CAD build for the part. Positions are in the model's coordinates, mm. A direction names the side the tool comes from. Round coordinates to 2 decimals unless told otherwise and drop trailing zeros. Order: outer loops, then holes, each group sorted by start corner. A loop starts at its lowest first (then second) coordinate and runs counter-clockwise, first axis right, second up. Notation, with made-up numbers: (-24, 77) - (14, 77) arc R14 cw to (14, 82) - close; hole circle Ø10 at (80.25, 87). An arc over 180 degrees is marked (long way). Write item = value, one per line.
from build123d import *

# Parameters (mm, degrees)
BOSS_EXTRUDE1_DEPTH = 20
SKETCH2_W           = 40
SKETCH2_H           = 40
BOSS_EXTRUDE2_DEPTH = 80
SKETCH3_W           = 40
SKETCH3_H           = 60
SKETCH3_H_2         = 40
SKETCH3_W_2         = 60
BOSS_EXTRUDE3_DEPTH = 20
SKETCH5_R           = 2.75
CUT_EXTRUDE1_DEPTH  = 167
FILLET1_R           = 25
FILLET2_R           = 15
SKETCH6_W           = 5
SKETCH6_H           = 10
SKETCH6_W_2         = 10
SKETCH6_H_2         = 5
BOSS_EXTRUDE4_DEPTH = 10
CUT_EXTRUDE2_DEPTH  = 10
CUT_EXTRUDE3_DEPTH  = 10
SKETCH9_W           = 10
SKETCH9_H           = 5
SKETCH9_W_2         = 5
SKETCH9_H_2         = 10
BOSS_EXTRUDE5_DEPTH = 10
CUT_EXTRUDE4_DEPTH  = 10
CUT_EXTRUDE5_DEPTH  = 10
FILLET4_R           = 3


with BuildPart() as part:
    # Sketch1 → Boss-Extrude1 (new body)
    with BuildSketch(Plane.XY):
        Polygon((100, 380), (100, 340), (40, 340), (40, 280), (0, 280), (0, 380), align=None)
    extrude(amount=BOSS_EXTRUDE1_DEPTH)

    # Sketch2 → Boss-Extrude2 (add)
    with BuildSketch(Plane.XY.offset(20)):
        with Locations((20, 360)):
            Rectangle(SKETCH2_W, SKETCH2_H)
    extrude(amount=BOSS_EXTRUDE2_DEPTH)

    # Sketch3 → Boss-Extrude3 (add)
    with BuildSketch(Plane.XY.offset(100)):
        with Locations((20, 310)):
            Rectangle(SKETCH3_W, SKETCH3_H)
        with Locations((20, 360)):
            Rectangle(SKETCH3_W, SKETCH3_H_2)
        with Locations((70, 360)):
            Rectangle(SKETCH3_W_2, SKETCH3_H_2)
    extrude(amount=BOSS_EXTRUDE3_DEPTH)

    # Sketch5 → Cut-Extrude1 (cut)
    with BuildSketch(Plane.XY.offset(120)):
        with Locations((55, 360)):
            Circle(SKETCH5_R)
        with BuildLine():
            ThreePointArc((82.25, 360), (85, 357.25), (87.75, 360))
            Line((87.75, 360), (82.25, 360))
        make_face()
        with BuildLine():
            Line((82.25, 360), (87.75, 360))
            ThreePointArc((87.75, 360), (85, 362.75), (82.25, 360))
        make_face()
        with Locations((20, 325)):
            Circle(SKETCH5_R)
        with BuildLine():
            ThreePointArc((22.75, 295), (21.944543648, 296.944543648), (20, 297.75))
            Line((20, 297.75), (20, 292.25))
            ThreePointArc((20, 292.25), (21.944543648, 293.055456352), (22.75, 295))
        make_face()
        with BuildLine():
            Line((20, 292.25), (20, 297.75))
            ThreePointArc((20, 297.75), (17.25, 295), (20, 292.25))
        make_face()
    extrude(amount=-CUT_EXTRUDE1_DEPTH, mode=Mode.SUBTRACT)

    # Fillet1
    # the kernel refuses this fillet: 25 mm, written as the material it takes off along each edge
    with BuildSketch(Plane(origin=(40, 340, 20), x_dir=(0, 1, 0), z_dir=(0, 0, 1))) as fillet1_piece_1:
        with BuildLine():
            CenterArc((FILLET1_R, FILLET1_R), FILLET1_R, 180, 90)
            Line((0, FILLET1_R), (0, 0))
            Line((0, 0), (FILLET1_R, 0))
        make_face()
    extrude(amount=80, mode=Mode.SUBTRACT)

    # Fillet2
    fillet2_edges = [part.edges().sort_by_distance(p)[0] for p in [
        (100, 340, 10),
        (40, 340, 10),
        (40, 280, 10),
        (40, 280, 110),
        (40, 340, 110),
        (100, 340, 110),
    ]]
    fillet(fillet2_edges, radius=FILLET2_R)

    # Sketch6 → Boss-Extrude4 (add)
    with BuildSketch(Plane.XY.offset(20)):
        with Locations((2.5, 310)):
            Rectangle(SKETCH6_W, SKETCH6_H)
        with Locations((70, 377.5)):
            Rectangle(SKETCH6_W_2, SKETCH6_H_2)
    extrude(amount=BOSS_EXTRUDE4_DEPTH)

    # Sketch7 → Cut-Extrude2 (cut)
    with BuildSketch(Plane.XZ.offset(-375)):
        with BuildLine():
            ThreePointArc((71.75, 25), (71.237436867, 26.237436867), (70, 26.75))
            Line((70, 26.75), (70, 23.25))
            ThreePointArc((70, 23.25), (71.237436867, 23.762563133), (71.75, 25))
        make_face()
        with BuildLine():
            Line((70, 23.25), (70, 26.75))
            ThreePointArc((70, 26.75), (68.25, 25), (70, 23.25))
        make_face()
    extrude(amount=-CUT_EXTRUDE2_DEPTH, mode=Mode.SUBTRACT)

    # Sketch8 → Cut-Extrude3 (cut)
    with BuildSketch(Plane(origin=(5, 0, 0), x_dir=(0, 0, -1), z_dir=(1, 0, 0))):
        with BuildLine():
            ThreePointArc((-23.25, 310), (-25, 311.75), (-26.75, 310))
            Line((-26.75, 310), (-23.25, 310))
        make_face()
        with BuildLine():
            Line((-23.25, 310), (-26.75, 310))
            ThreePointArc((-26.75, 310), (-25, 308.25), (-23.25, 310))
        make_face()
    extrude(amount=-CUT_EXTRUDE3_DEPTH, mode=Mode.SUBTRACT)

    # Sketch9 → Boss-Extrude5 (add)
    with BuildSketch(Plane(origin=(0, 0, 100), x_dir=(-1, 0, 0), z_dir=(0, 0, -1))):
        with Locations((-70, 377.5)):
            Rectangle(SKETCH9_W, SKETCH9_H)
        with Locations((-2.5, 310)):
            Rectangle(SKETCH9_W_2, SKETCH9_H_2)
    extrude(amount=BOSS_EXTRUDE5_DEPTH)

    # Sketch10 → Cut-Extrude4 (cut)
    with BuildSketch(Plane(origin=(5, 0, 0), x_dir=(0, 0, -1), z_dir=(1, 0, 0))):
        with BuildLine():
            ThreePointArc((-96.75, 310), (-95, 308.25), (-93.25, 310))
            Line((-93.25, 310), (-96.75, 310))
        make_face()
        with BuildLine():
            Line((-96.75, 310), (-93.25, 310))
            ThreePointArc((-93.25, 310), (-95, 311.75), (-96.75, 310))
        make_face()
    extrude(amount=-CUT_EXTRUDE4_DEPTH, mode=Mode.SUBTRACT)

    # Sketch11 → Cut-Extrude5 (cut)
    with BuildSketch(Plane.XZ.offset(-375)):
        with BuildLine():
            ThreePointArc((71.75, 95), (71.237436867, 96.237436867), (70, 96.75))
            Line((70, 96.75), (70, 93.25))
            ThreePointArc((70, 93.25), (71.237436867, 93.762563133), (71.75, 95))
        make_face()
        with BuildLine():
            Line((70, 93.25), (70, 96.75))
            ThreePointArc((70, 96.75), (68.25, 95), (70, 93.25))
        make_face()
    extrude(amount=-CUT_EXTRUDE5_DEPTH, mode=Mode.SUBTRACT)

    # Fillet4
    fillet4_edges = [part.edges().sort_by_distance(p)[0] for p in [
        (2.5, 315, 30),
        (2.5, 305, 20),
        (2.5, 305, 30),
        (2.5, 315, 20),
        (75, 377.5, 30),
        (65, 377.5, 20),
        (65, 377.5, 30),
        (75, 377.5, 20),
        (65, 377.5, 100),
        (75, 377.5, 100),
        (65, 377.5, 90),
        (75, 377.5, 90),
        (2.5, 305, 100),
        (2.5, 315, 100),
        (2.5, 305, 90),
        (2.5, 315, 90),
    ]]
    fillet(fillet4_edges, radius=FILLET4_R)


solid = part.part
(1) Tool access for faces 1 (the cylindrical face through (2.54, 305.86, 29.1)), 2 (the cylindrical face through (32.482, 347.129, 59.44)), 3 (the flat face through (70, 378, 30)), 4 (the cylindrical face through (64.1, 377.54, 99.14)): list every direction of +Z, -Z, +X, -X, +Y, -Y with a clear straight run to the whole face (end or side of a thin tool).
Solved:
face_1 = +X, -X, -Y
face_2 = +X, -Y
face_3 = +X, +Y, -Y
face_4 = +Y, -Y
(2) Band-saw the part on A-A on z = 106. List the corners of the cut face in (x, y).
Solved:
outline = (0, 280) - (25, 280) arc R15 ccw to (40, 295) - (40, 325) arc R15 cw to (55, 340) - (85, 340) arc R15 ccw to (100, 355) - (100, 380) - (0, 380) - close; hole circle Ø5.5 at (20, 295); hole circle Ø5.5 at (20, 325); hole circle Ø5.5 at (55, 360); hole circle Ø5.5 at (85, 360)
(3) Drop flat-ended pins along their axis: pin 1 (4 mm diameter, centred on y = 315.5, z = 93, fed in from +X); pin 2 (7.5 mm diameter, centred on y = 375, z = 71, fed in from +X); pin 3 (2 mm diameter, centred on x = 69, y = 378, fed in from -Z); pin 4 (6 mm diameter, centred on x = 67, z = 6, fed in from -Y). Give the stop position or say it passes through.
Solved:
pin_1 = 5
pin_2 = 40
pin_3 = 0
pin_4 = 340
(4) Band-saw the part on B-B on y = 310. List the corners of the cut face in (x, z), plus the area to 4 significant figures.
Solved:
outline = (0, 0) - (40, 0) - (40, 20) - (5, 20) - (5, 23.25) - (0, 23.25) - close; (0, 26.75) - (5, 26.75) - (5, 30) - (0, 30) - close; (0, 90) - (5, 90) - (5, 93.25) - (0, 93.25) - close; (0, 96.75) - (5, 96.75) - (5, 100) - (40, 100) - (40, 120) - (0, 120) - close
area = 1,665 mm²
(5) Pull direction Y, two halves, no side cores. Call faces 5 (the flat face through (70, 340, 10)), 6 (the cylindrical face through (2.54, 311.71, 24.62)), 7 (the flat face through (100, 368, 10)): released by +Y, released by -Y, zero draft, split by the parting line, or undercut.
Solved:
face_5 = released by -Y
face_6 = undercut
face_7 = zero draft
(6) Band-saw the part on C-C on z = 77. List the corners of the cut face in (x, y), plus the area to 3 significant figures.
Solved:
outline = (0, 340) - (15, 340) arc R25 ccw to (40, 365) - (40, 380) - (0, 380) - close
area = 1,470 mm²
(7) Band-saw the part on D-D on y = 290.5. List the corners of the cut face in (x, z).
Solved:
outline = (0, 0) - (39.31, 0) - (39.31, 20) - (0, 20) - close; (0, 100) - (39.31, 100) - (39.31, 120) - (0, 120) - close
(8) Probe line 1 along Z through (x, y) = (1.2, 310); line 2 along X through (y, z) = (360, 106.25); line 3 along Z through (x, y) = (75, 351). List the from-to ranges inside material, lowest first.
Solved:
line_1 = 0 to 23.25, 26.75 to 30, 90 to 93.25, 96.75 to 120
line_2 = 0 to 52.25, 57.75 to 82.25, 87.75 to 100
line_3 = 0 to 20, 100 to 120
